Can you work these out from the drawing? Everything is in mm from the part's minimum corner. A direction names the side the tool comes from. Coordinates: 2 decimals unless noted, no trailing zeros. Write each loop counter-clockwise with the first axis right and the second up, starting at its lowest first coordinate (ties: lowest second). Pieces come first, ordered by that corner, then holes.
(1) Which directions (+Z, -Z, +X, -X, +Y, -Y) give clear straight access to the entire face, cutting with the end or side of a thin tool? Please do the marked faces 4 and 5.
(2) Imagine slicing it at B-B, the plane z = 10. List the corners of the cut face in (x, y) for me, plus the area to 3 significant figures.
(3) For pin 1 Ø8 at (y, z) = (7.5, 10) entering from +X, with a flat end and sliding along its axis, tell me the tip position at first contact or that it passes through.
(4) Thinking about a two-plate mould opening in Y: for the marked faces 1, 2 and 3, which applies, released by +Y, released by -Y, zero draft, split by the parting line, or undercut?
(5) Imagine slicing it at C-C, the plane y = 5.25. List the corners of the cut face in (x, z) for me, plus the area to 3 significant figures.
(6) Imagine slicing it at D-D, the plane x = 3.95. List the corners of the cut face in (y, z) for me.
(7) Please list where these lines run through material, in increasing order: probe 1 along Y at (x, z) = (2.85, 10); probe 2 along Y at (x, z) = (4.85, 7.5); probe 3 along Z at (x, y) = (4.7, 10.75).
(8) Imagine slicing it at A-A, the plane x = 0.75. List the corners of the cut face in (y, z) for me, plus the area to 3 significant figures.
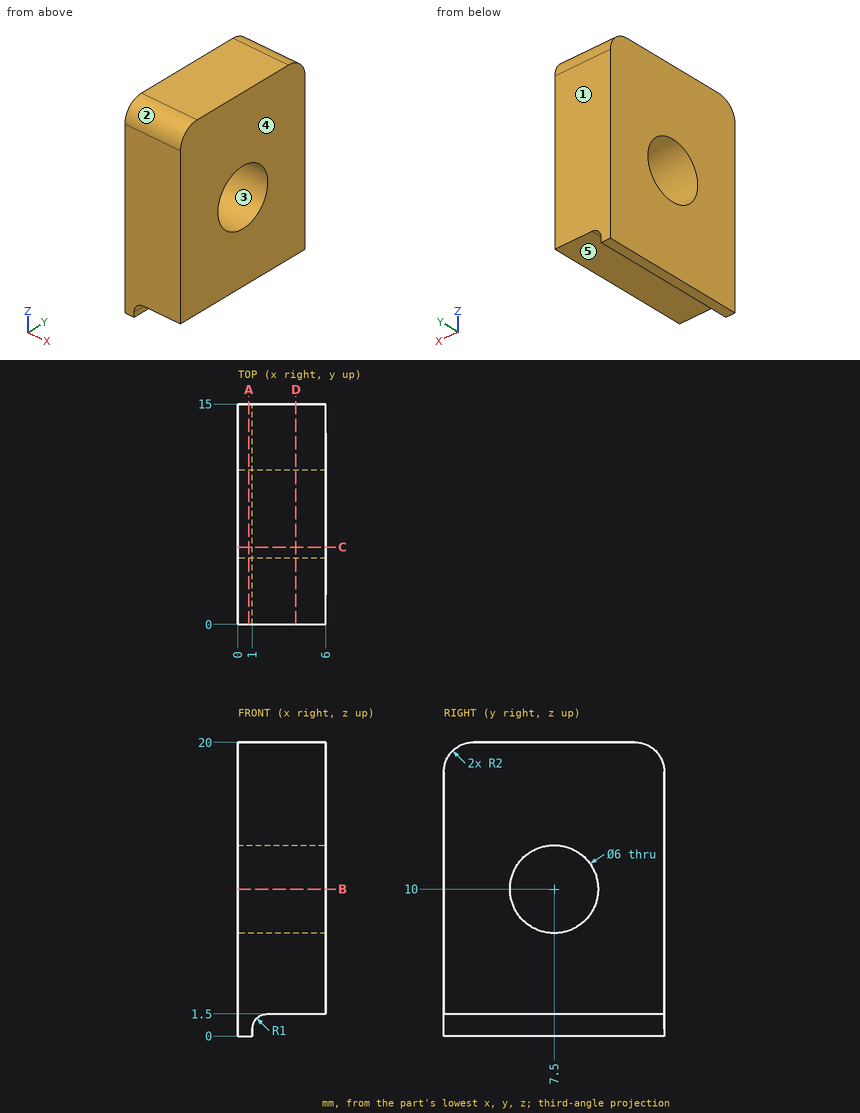
Recorded:
1. face 4: +Z, -Z, +X, +Y, -Y
1. face 5: -Z, +X, +Y, -Y
2. outline: (0, 0) - (6, 0) - (6, 4.5) - (0, 4.5) - close; (0, 10.5) - (6, 10.5) - (6, 15) - (0, 15) - close
2. area: 54.0 mm2
3. pin 1: stops at x = 6
4. face 1: released by +Y
4. face 2: released by -Y
4. face 3: undercut
5. outline: (0, 0) - (1, 0) - (1, 0.5) arc R1 cw to (2, 1.5) - (6, 1.5) - (6, 8.02) - (0, 8.02) - close; (0, 11.98) - (6, 11.98) - (6, 20) - (0, 20) - close
5. area: 88.9 mm2
6. outline: (0, 1.5) - (15, 1.5) - (15, 18) arc R2 ccw to (13, 20) - (2, 20) arc R2 ccw to (0, 18) - close; hole circle Ø6 at (7.5, 10)
7. probe 1: y = 0 to 4.5, 10.5 to 15
7. probe 2: y = 0 to 5.84, 9.16 to 15
7. probe 3: z = 1.5 to 20
8. outline: (0, 0) - (15, 0) - (15, 18) arc R2 ccw to (13, 20) - (2, 20) arc R2 ccw to (0, 18) - close; hole circle Ø6 at (7.5, 10)
8. area: 270 mm2
